Verification items for the finished model (mm, model axes). Coordinates: 2 decimals unless noted, no trailing zeros. Order: outer loops, then holes, each group sorted by start corner. A loop starts at its lowest first (then second) coordinate and runs counter-clockwise, first axis right, second up. Notation, with made-up numbers: M 52.25,2 L 56.25,2 A25 cw 56.25,18 Z; hole C 20,-23.75 d6. An arc over 180 degrees is marked long. Write item = value, one per line.
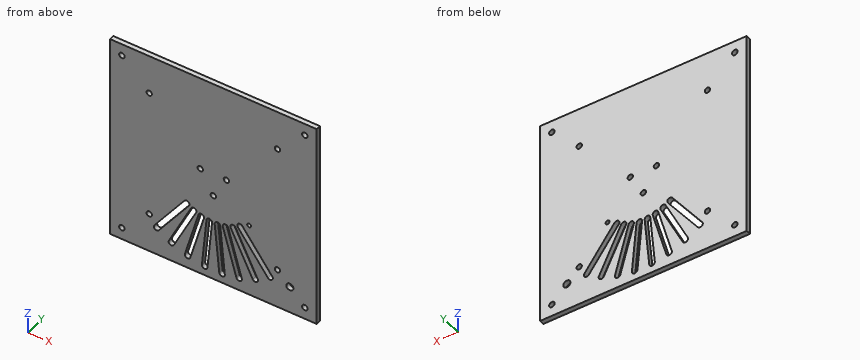
```python
from build123d import *

# Parameters (mm, degrees)
SKETCH2_W                 = 130
SKETCH2_H                 = 130
BOSS_EXTRUDE1_DEPTH       = 3
CORNERPIECE_HOLES_REACH   = 93.973
SKETCH4_R                 = 1.75
CUT_EXTRUDE2_REACH        = 93.973
SKETCH6_R                 = 1.7
CUT_EXTRUDE3_REACH        = 93.973
SKETCH8_R                 = 1.7
PRIMARY_WIRE_HOLE_REACH   = 93.973
SKETCH9_R                 = 2.25
SECONDARY_WIRE_HOLE_REACH = 93.973
SKETCH10_R                = 1.25
CUT_EXTRUDE6_REACH        = 93.973


with BuildPart() as part:
    # Sketch2 → Boss-Extrude1 (new body)
    with BuildSketch(Plane(origin=(0, 0, 0), x_dir=(1, 0, 0), z_dir=(0, 1, 0))):
        Rectangle(SKETCH2_W, SKETCH2_H)
    extrude(amount=BOSS_EXTRUDE1_DEPTH)

    # Sketch4 → Cornerpiece holes (cut, up to next)
    with BuildSketch(Plane(origin=(0, 3, 0), x_dir=(1, 0, 0), z_dir=(0, 1, 0)), mode=Mode.PRIVATE) as cornerpiece_holes_sk1:
        with Locations(Location((-57.5, 57.5, 0), (0, 0, 270))):
            Circle(SKETCH4_R)
    cornerpiece_holes_tool1 = extrude(cornerpiece_holes_sk1.sketch, amount=-CORNERPIECE_HOLES_REACH, mode=Mode.PRIVATE) & part.part
    # Sketch4 → Cornerpiece holes (cut, up to next)
    with BuildSketch(Plane(origin=(0, 3, 0), x_dir=(1, 0, 0), z_dir=(0, 1, 0)), mode=Mode.PRIVATE) as cornerpiece_holes_sk2:
        with Locations(Location((57.5, 57.5, 0), (0, 0, 270))):
            Circle(SKETCH4_R)
    cornerpiece_holes_tool2 = extrude(cornerpiece_holes_sk2.sketch, amount=-CORNERPIECE_HOLES_REACH, mode=Mode.PRIVATE) & part.part
    # Sketch4 → Cornerpiece holes (cut, up to next)
    with BuildSketch(Plane(origin=(0, 3, 0), x_dir=(1, 0, 0), z_dir=(0, 1, 0)), mode=Mode.PRIVATE) as cornerpiece_holes_sk3:
        with Locations(Location((57.5, -57.5, 0), (0, 0, 270))):
            Circle(SKETCH4_R)
    cornerpiece_holes_tool3 = extrude(cornerpiece_holes_sk3.sketch, amount=-CORNERPIECE_HOLES_REACH, mode=Mode.PRIVATE) & part.part
    # Sketch4 → Cornerpiece holes (cut, up to next)
    with BuildSketch(Plane(origin=(0, 3, 0), x_dir=(1, 0, 0), z_dir=(0, 1, 0)), mode=Mode.PRIVATE) as cornerpiece_holes_sk4:
        with Locations(Location((-57.5, -57.5, 0), (0, 0, 270))):
            Circle(SKETCH4_R)
    cornerpiece_holes_tool4 = extrude(cornerpiece_holes_sk4.sketch, amount=-CORNERPIECE_HOLES_REACH, mode=Mode.PRIVATE) & part.part
    add(cornerpiece_holes_tool1.solids().sort_by_distance((-57.5, 3, -57.5))[0], mode=Mode.SUBTRACT)
    add(cornerpiece_holes_tool2.solids().sort_by_distance((57.5, 3, -57.5))[0], mode=Mode.SUBTRACT)
    add(cornerpiece_holes_tool3.solids().sort_by_distance((57.5, 3, 57.5))[0], mode=Mode.SUBTRACT)
    add(cornerpiece_holes_tool4.solids().sort_by_distance((-57.5, 3, 57.5))[0], mode=Mode.SUBTRACT)

    # Sketch6 → Cut-Extrude2 (cut, up to next)
    with BuildSketch(Plane(origin=(0, 3, 0), x_dir=(1, 0, 0), z_dir=(0, 1, 0)), mode=Mode.PRIVATE) as cut_extrude2_sk1:
        with Locations(Location((-40.305086528, 40.305086528, 0), (0, 0, 270))):
            Circle(SKETCH6_R)
    cut_extrude2_tool1 = extrude(cut_extrude2_sk1.sketch, amount=-CUT_EXTRUDE2_REACH, mode=Mode.PRIVATE) & part.part
    # Sketch6 → Cut-Extrude2 (cut, up to next)
    with BuildSketch(Plane(origin=(0, 3, 0), x_dir=(1, 0, 0), z_dir=(0, 1, 0)), mode=Mode.PRIVATE) as cut_extrude2_sk2:
        with Locations(Location((40.305086528, 40.305086528, 0), (0, 0, 270))):
            Circle(SKETCH6_R)
    cut_extrude2_tool2 = extrude(cut_extrude2_sk2.sketch, amount=-CUT_EXTRUDE2_REACH, mode=Mode.PRIVATE) & part.part
    # Sketch6 → Cut-Extrude2 (cut, up to next)
    with BuildSketch(Plane(origin=(0, 3, 0), x_dir=(1, 0, 0), z_dir=(0, 1, 0)), mode=Mode.PRIVATE) as cut_extrude2_sk3:
        with Locations(Location((40.305086528, -40.305086528, 0), (0, 0, 270))):
            Circle(SKETCH6_R)
    cut_extrude2_tool3 = extrude(cut_extrude2_sk3.sketch, amount=-CUT_EXTRUDE2_REACH, mode=Mode.PRIVATE) & part.part
    # Sketch6 → Cut-Extrude2 (cut, up to next)
    with BuildSketch(Plane(origin=(0, 3, 0), x_dir=(1, 0, 0), z_dir=(0, 1, 0)), mode=Mode.PRIVATE) as cut_extrude2_sk4:
        with Locations(Location((-40.305086528, -40.305086528, 0), (0, 0, 270))):
            Circle(SKETCH6_R)
    cut_extrude2_tool4 = extrude(cut_extrude2_sk4.sketch, amount=-CUT_EXTRUDE2_REACH, mode=Mode.PRIVATE) & part.part
    add(cut_extrude2_tool1.solids().sort_by_distance((-40.305087, 3, -40.305087))[0], mode=Mode.SUBTRACT)
    add(cut_extrude2_tool2.solids().sort_by_distance((40.305087, 3, -40.305087))[0], mode=Mode.SUBTRACT)
    add(cut_extrude2_tool3.solids().sort_by_distance((40.305087, 3, 40.305087))[0], mode=Mode.SUBTRACT)
    add(cut_extrude2_tool4.solids().sort_by_distance((-40.305087, 3, 40.305087))[0], mode=Mode.SUBTRACT)

    # Sketch8 → Cut-Extrude3 (cut, up to next)
    with BuildSketch(Plane(origin=(0, 3, 0), x_dir=(1, 0, 0), z_dir=(0, 1, 0)), mode=Mode.PRIVATE) as cut_extrude3_sk1:
        with Locations(Location((0, 9.5, 0), (0, 0, 270))):
            Circle(SKETCH8_R)
    cut_extrude3_tool1 = extrude(cut_extrude3_sk1.sketch, amount=-CUT_EXTRUDE3_REACH, mode=Mode.PRIVATE) & part.part
    # Sketch8 → Cut-Extrude3 (cut, up to next)
    with BuildSketch(Plane(origin=(0, 3, 0), x_dir=(1, 0, 0), z_dir=(0, 1, 0)), mode=Mode.PRIVATE) as cut_extrude3_sk2:
        with Locations(Location((8.227241336, -4.75, 0), (0, 0, 270))):
            Circle(SKETCH8_R)
    cut_extrude3_tool2 = extrude(cut_extrude3_sk2.sketch, amount=-CUT_EXTRUDE3_REACH, mode=Mode.PRIVATE) & part.part
    # Sketch8 → Cut-Extrude3 (cut, up to next)
    with BuildSketch(Plane(origin=(0, 3, 0), x_dir=(1, 0, 0), z_dir=(0, 1, 0)), mode=Mode.PRIVATE) as cut_extrude3_sk3:
        with Locations(Location((-8.227241336, -4.75, 0), (0, 0, 270))):
            Circle(SKETCH8_R)
    cut_extrude3_tool3 = extrude(cut_extrude3_sk3.sketch, amount=-CUT_EXTRUDE3_REACH, mode=Mode.PRIVATE) & part.part
    add(cut_extrude3_tool1.solids().sort_by_distance((0, 3, -9.5))[0], mode=Mode.SUBTRACT)
    add(cut_extrude3_tool2.solids().sort_by_distance((8.227241, 3, 4.75))[0], mode=Mode.SUBTRACT)
    add(cut_extrude3_tool3.solids().sort_by_distance((-8.227241, 3, 4.75))[0], mode=Mode.SUBTRACT)

    # Sketch9 → Primary wire hole (cut, up to next)
    with BuildSketch(Plane(origin=(0, 3, 0), x_dir=(1, 0, 0), z_dir=(0, 1, 0)), mode=Mode.PRIVATE) as primary_wire_hole_sk1:
        with Locations(Location((48.083261121, 48.083261121, 0), (0, 0, 270))):
            Circle(SKETCH9_R)
    primary_wire_hole_tool1 = extrude(primary_wire_hole_sk1.sketch, amount=-PRIMARY_WIRE_HOLE_REACH, mode=Mode.PRIVATE) & part.part
    add(primary_wire_hole_tool1.solids().sort_by_distance((48.083261, 3, -48.083261))[0], mode=Mode.SUBTRACT)

    # Sketch10 → Secondary wire hole (cut, up to next)
    with BuildSketch(Plane(origin=(0, 3, 0), x_dir=(1, 0, 0), z_dir=(0, 1, 0)), mode=Mode.PRIVATE) as secondary_wire_hole_sk1:
        with Locations(Location((22.506385739, 18.885099973, 0), (0, 0, 270))):
            Circle(SKETCH10_R)
    secondary_wire_hole_tool1 = extrude(secondary_wire_hole_sk1.sketch, amount=-SECONDARY_WIRE_HOLE_REACH, mode=Mode.PRIVATE) & part.part
    add(secondary_wire_hole_tool1.solids().sort_by_distance((22.506386, 3, -18.8851))[0], mode=Mode.SUBTRACT)

    # Sketch11 → Cut-Extrude6 (cut, up to next)
    with BuildSketch(Plane(origin=(0, 3, 0), x_dir=(1, 0, 0), z_dir=(0, 1, 0)), mode=Mode.PRIVATE) as cut_extrude6_sk1:
        with BuildLine():
            Line((-34.259927979, 48.372330261), (-15.380990703, 23.319134311))
            ThreePointArc((-15.380990703, 23.319134311), (-15.725426555, 20.868345878), (-18.176214988, 21.21278173))
            Line((-18.176214988, 21.21278173), (-37.055152264, 46.26597768))
            ThreePointArc((-37.055152264, 46.26597768), (-36.710716412, 48.716766113), (-34.259927979, 48.372330261))
        make_face()
    cut_extrude6_tool1 = extrude(cut_extrude6_sk1.sketch, amount=-CUT_EXTRUDE6_REACH, mode=Mode.PRIVATE) & part.part
    # Sketch11 → Cut-Extrude6 (cut, up to next)
    with BuildSketch(Plane(origin=(0, 3, 0), x_dir=(1, 0, 0), z_dir=(0, 1, 0)), mode=Mode.PRIVATE) as cut_extrude6_sk2:
        with BuildLine():
            Line((-27.938203096, 52.278884913), (-13.975987518, 24.187365977))
            ThreePointArc((-13.975987518, 24.187365977), (-11.629987027, 23.399151731), (-10.841772782, 25.745152222))
            Line((-10.841772782, 25.745152222), (-24.80398836, 53.836671159))
            ThreePointArc((-24.80398836, 53.836671159), (-27.149988851, 54.624885404), (-27.938203096, 52.278884913))
        make_face()
    cut_extrude6_tool2 = extrude(cut_extrude6_sk2.sketch, amount=-CUT_EXTRUDE6_REACH, mode=Mode.PRIVATE) & part.part
    # Sketch11 → Cut-Extrude6 (cut, up to next)
    with BuildSketch(Plane(origin=(0, 3, 0), x_dir=(1, 0, 0), z_dir=(0, 1, 0)), mode=Mode.PRIVATE) as cut_extrude6_sk3:
        with BuildLine():
            Line((-17.87286129, 56.517128637), (-9.301329978, 26.340883824))
            ThreePointArc((-9.301329978, 26.340883824), (-7.139754963, 25.135647974), (-5.934519112, 27.297222989))
            Line((-5.934519112, 27.297222989), (-14.506050425, 57.473467801))
            ThreePointArc((-14.506050425, 57.473467801), (-16.667625439, 58.678703651), (-17.87286129, 56.517128637))
        make_face()
    cut_extrude6_tool3 = extrude(cut_extrude6_sk3.sketch, amount=-CUT_EXTRUDE6_REACH, mode=Mode.PRIVATE) & part.part
    # Sketch11 → Cut-Extrude6 (cut, up to next)
    with BuildSketch(Plane(origin=(0, 3, 0), x_dir=(1, 0, 0), z_dir=(0, 1, 0)), mode=Mode.PRIVATE) as cut_extrude6_sk4:
        with BuildLine():
            Line((-7.200805802, 58.836837065), (-4.310928692, 27.600231771))
            ThreePointArc((-4.310928692, 27.600231771), (-2.407156164, 26.018887355), (-0.825811748, 27.922659883))
            Line((-0.825811748, 27.922659883), (-3.715688858, 59.159265177))
            ThreePointArc((-3.715688858, 59.159265177), (-5.619461386, 60.740609593), (-7.200805802, 58.836837065))
        make_face()
    cut_extrude6_tool4 = extrude(cut_extrude6_sk4.sketch, amount=-CUT_EXTRUDE6_REACH, mode=Mode.PRIVATE) & part.part
    # Sketch11 → Cut-Extrude6 (cut, up to next)
    with BuildSketch(Plane(origin=(0, 3, 0), x_dir=(1, 0, 0), z_dir=(0, 1, 0)), mode=Mode.PRIVATE) as cut_extrude6_sk5:
        with BuildLine():
            Line((3.715688858, 59.159265177), (0.825811748, 27.922659883))
            ThreePointArc((0.825811748, 27.922659883), (2.407156164, 26.018887355), (4.310928692, 27.600231771))
            Line((4.310928692, 27.600231771), (7.200805802, 58.836837065))
            ThreePointArc((7.200805802, 58.836837065), (5.619461386, 60.740609593), (3.715688858, 59.159265177))
        make_face()
    cut_extrude6_tool5 = extrude(cut_extrude6_sk5.sketch, amount=-CUT_EXTRUDE6_REACH, mode=Mode.PRIVATE) & part.part
    # Sketch11 → Cut-Extrude6 (cut, up to next)
    with BuildSketch(Plane(origin=(0, 3, 0), x_dir=(1, 0, 0), z_dir=(0, 1, 0)), mode=Mode.PRIVATE) as cut_extrude6_sk6:
        with BuildLine():
            Line((14.506050425, 57.473467801), (5.934519112, 27.297222989))
            ThreePointArc((5.934519112, 27.297222989), (7.139754963, 25.135647974), (9.301329978, 26.340883824))
            Line((9.301329978, 26.340883824), (17.87286129, 56.517128637))
            ThreePointArc((17.87286129, 56.517128637), (16.667625439, 58.678703651), (14.506050425, 57.473467801))
        make_face()
    cut_extrude6_tool6 = extrude(cut_extrude6_sk6.sketch, amount=-CUT_EXTRUDE6_REACH, mode=Mode.PRIVATE) & part.part
    # Sketch11 → Cut-Extrude6 (cut, up to next)
    with BuildSketch(Plane(origin=(0, 3, 0), x_dir=(1, 0, 0), z_dir=(0, 1, 0)), mode=Mode.PRIVATE) as cut_extrude6_sk7:
        with BuildLine():
            Line((24.80398836, 53.836671159), (10.841772782, 25.745152222))
            ThreePointArc((10.841772782, 25.745152222), (11.629987027, 23.399151731), (13.975987518, 24.187365977))
            Line((13.975987518, 24.187365977), (27.938203096, 52.278884913))
            ThreePointArc((27.938203096, 52.278884913), (27.149988851, 54.624885404), (24.80398836, 53.836671159))
        make_face()
    cut_extrude6_tool7 = extrude(cut_extrude6_sk7.sketch, amount=-CUT_EXTRUDE6_REACH, mode=Mode.PRIVATE) & part.part
    # Sketch11 → Cut-Extrude6 (cut, up to next)
    with BuildSketch(Plane(origin=(0, 3, 0), x_dir=(1, 0, 0), z_dir=(0, 1, 0)), mode=Mode.PRIVATE) as cut_extrude6_sk8:
        with BuildLine():
            Line((34.259927979, 48.372330261), (15.380990703, 23.319134311))
            ThreePointArc((15.380990703, 23.319134311), (15.725426555, 20.868345878), (18.176214988, 21.21278173))
            Line((18.176214988, 21.21278173), (37.055152264, 46.26597768))
            ThreePointArc((37.055152264, 46.26597768), (36.710716412, 48.716766113), (34.259927979, 48.372330261))
        make_face()
    cut_extrude6_tool8 = extrude(cut_extrude6_sk8.sketch, amount=-CUT_EXTRUDE6_REACH, mode=Mode.PRIVATE) & part.part
    add(cut_extrude6_tool1.solids().sort_by_distance((-26.218071, 3, -34.792556))[0], mode=Mode.SUBTRACT)
    add(cut_extrude6_tool2.solids().sort_by_distance((-19.389988, 3, -39.012019))[0], mode=Mode.SUBTRACT)
    add(cut_extrude6_tool3.solids().sort_by_distance((-11.90369, 3, -41.907176))[0], mode=Mode.SUBTRACT)
    add(cut_extrude6_tool4.solids().sort_by_distance((-4.013309, 3, -43.379748))[0], mode=Mode.SUBTRACT)
    add(cut_extrude6_tool5.solids().sort_by_distance((4.013309, 3, -43.379748))[0], mode=Mode.SUBTRACT)
    add(cut_extrude6_tool6.solids().sort_by_distance((11.90369, 3, -41.907176))[0], mode=Mode.SUBTRACT)
    add(cut_extrude6_tool7.solids().sort_by_distance((19.389988, 3, -39.012019))[0], mode=Mode.SUBTRACT)
    add(cut_extrude6_tool8.solids().sort_by_distance((26.218071, 3, -34.792556))[0], mode=Mode.SUBTRACT)


solid = part.part
```
Item 1: Gauge pin test, flat end, axial feed: pin 1 (2 mm diameter, centred on x = 40.31, z = 40.31, fed in from +Y). Record the tip position at first contact, or that the pin passes through.
Report:
pin_1 = through
Item 2: Sectioned sample at C-C, the plane z = -9.5. Enter the section's corners in (x, y).
Report:
outline = M -65,0 L -1.7,0 L -1.7,3 L -65,3 Z; M 1.7,0 L 65,0 L 65,3 L 1.7,3 Z
Item 3: Sectioned sample at D-D, the plane y = 1.6. Give the number of separate pieces and of enclosed holes in the cut face, then the cut area to 3 significant figures.
Report:
separate_pieces = 1
enclosed_holes = 21
area = 15,800 mm^2
Item 4: Sectioned sample at B-B, the plane x = 57.5. Enter the section's corners in (y, z), then the cut area to 3 significant figures.
Report:
outline = M 0,-65 L 3,-65 L 3,-59.25 L 0,-59.25 Z; M 0,-55.75 L 3,-55.75 L 3,55.75 L 0,55.75 Z; M 0,59.25 L 3,59.25 L 3,65 L 0,65 Z
area = 369 mm^2
Item 5: Sectioned sample at A-A, the plane z = 4.75. Enter the section's corners in (x, y).
Report:
outline = M -65,0 L -9.93,0 L -9.93,3 L -65,3 Z; M -6.53,0 L 6.53,0 L 6.53,3 L -6.53,3 Z; M 9.93,0 L 65,0 L 65,3 L 9.93,3 Z
Item 6: Scan lines: L1, parallel to X at y = 2.3, z = 57.5; L2, parallel to Z at x = -41, y = 2.25; L3, parallel to Z at x = -27, y = 1.7. Record each from-to range of solid material in increasing order. Write a range as from..to.
Report:
L1 = -65..-59.25, -55.75..55.75, 59.25..65
L2 = -65..-41.86, -38.75..38.75, 41.86..65
L3 = -65..-54.69, -50.39..-38.74, -32.92..65
